from build123d import *


with BuildPart() as part:
    # Эскиз2 → Повернуть1 (revolve)
    with BuildSketch(Plane(origin=(0, 0, 0), x_dir=(0, 0, -1), z_dir=(1, 0, 0))):
        with BuildLine():
            Line((10.5, 0), (10.5, 32))
            Line((10.5, 32), (12.5, 32))
            Line((12.5, 32), (12.5, 29.5))
            Line((12.5, 29.5), (19.944344329, 29.5))
            Line((19.944344329, 29.5), (23.412925951, 24.236876385))
            Line((23.412925951, 24.236876385), (48.626846206, 24.236876385))
            Line((48.626846206, 24.236876385), (56.389969821, 32))
            Line((56.389969821, 32), (71.909127128, 32))
            ThreePointArc((71.909127128, 32), (75.444661033, 30.535533906), (76.909127128, 27))
            Line((76.909127128, 27), (76.909127128, 5))
            ThreePointArc((76.909127128, 5), (75.444661033, 1.464466094), (71.909127128, 0))
            Line((71.909127128, 0), (56.389969821, 0))
            Line((56.389969821, 0), (48.643821993, 5.968581622))
            Line((48.643821993, 5.968581622), (23.412925951, 5.968581622))
            Line((23.412925951, 5.968581622), (19.944344329, 2.5))
            Line((19.944344329, 2.5), (12.5, 2.5))
            Line((12.5, 2.5), (12.5, 0))
            Line((12.5, 0), (10.5, 0))
        make_face()
    revolve(axis=Axis((0, 76.584186447, 0), (0, -1, 0)))


solid = part.part
Can you work these out from the model? Positions are in its coordinate system, mm. A direction names the side the tool comes from. Round coordinates to 2 decimals unless told otherwise and drop trailing zeros. Loops run counter-clockwise (first coordinate to the right, second up) from the corner with the lowest first, then second, coordinate; pieces in that order, holes last. Notation, with made-up numbers: (-9.75, 84) - (15.25, 84) arc R26 ccw to (15.25, 103) - close; hole circle Ø6 at (75, 39). An arc over 180 degrees is marked (long way). Answer in a Markdown table with one row per item. Add a question column.
Q1. Which directions (+Z, -Z, +X, -X, +Y, -Y) give clear straight access to the entire face, cutting with the end or side of a thin tool? Please do faces 5 (the flat face through (-37, 32, -43)), 6 (the cylindrical face through (3.755, 1.232, -11.923)), 7 (the flat face through (11, 24.237, 21)).
Q2. I want a section at A-A on y = 15.5. List the corners of the cut face in (x, z) for me.
Q3. For pin 1 Ø5 at (x, z) = (-36, -22) entering from +Y; pin 2 Ø1.5 at (x, y) = (-10, 25.5) entering from +Z; pin 3 Ø10 at (y, z) = (25, 18.5) entering from -X (3 decimals); pin 4 Ø19 at (x, z) = (0, 0) entering from -Y, each with a flat end and sliding along its axis, tell me the tip position at first contact or that it passes through.
Q4. I need wall thicknesses on L1, parallel to X at y = 18, z = 0; L2, parallel to X at y = 25, z = 0; L3, parallel to Y at x = -31, z = 16. Which ranges of each line are inside material? Lowest first, please.
Q5. We'd pull the mould along X, two halves only. Please class faces 1 (the flat face through (-37, 0, 43)), 2 (the cylindrical face through (23.1, 15.85, -73.36)), 3 (the conical face through (-19.634, 2.668, 4.36)), 4 (the cylindrical face through (3.2, 16.2, -10)): pulls with the +X half, pulls with the -X half, needs draft (parallel to the pull), parting line crosses it, or undercut.
A:
| question | item | result |
|---|---|---|
| 1 | face 5 | +Z, -Z, +X, -X, +Y |
| 1 | face 6 | -Y |
| 1 | face 7 | +Y |
| 2 | outline | circle Ø153.82 at (0, 0); hole circle Ø21 at (0, 0) |
| 3 | pin 1 | y = 24.24 |
| 3 | pin 2 | z = 76.35 |
| 3 | pin 3 | x = -75.715 |
| 3 | pin 4 | through |
| 4 | L1 | -76.91 to -10.5, 10.5 to 76.91 |
| 4 | L2 | -76.91 to -49.39, -22.91 to -10.5, 10.5 to 22.91, 49.39 to 76.91 |
| 4 | L3 | 5.97 to 24.24 |
| 5 | face 1 | needs draft |
| 5 | face 2 | parting line crosses it |
| 5 | face 3 | undercut |
| 5 | face 4 | undercut |
